Part model, mm, in its own coordinate system. Face numbers are marked on the shaded views. A direction names the side the tool comes from. Round coordinates to 2 decimals unless told otherwise and drop trailing zeros. Write each loop counter-clockwise with the first axis right and the second up, starting at its lowest first coordinate (ties: lowest second). Pieces come first, ordered by that corner, then holes.
1) Pull direction Y, two halves, no side cores. Call the marked faces 3, 4 and 5: +Y half, -Y half, draft (parallel to the pull), parting line (faces both ways), or undercut.
2) Saw through at A-A on y = 0. Write the cut outline in (x, z) (3 decimals).
3) Saw through at D-D on z = -30.5. Write the cut outline in (x, y) (3 decimals), and give its area (3 significant figures).
4) Which spindle directions (+Z, -Z, +X, -X, +Y, -Y) get a long thin tool onto all of the face, cutting with end or side? Do the marked faces 1 and 2. Say none if no direction does.
5) Drill centre lines: L1, parallel to Y at x = 0, z = 8.5 (3 decimals); L2, parallel to Y at x = 0, z = -36 (3 decimals); L3, parallel to Y at x = 1, z = -16. Where is each one in solid material? Low to high.
6) Saw through at B-B on x = 0. Write the cut outline in (y, z) (3 decimals).
7) Flat gauge pins, fed straight in: pin 1 (6 mm diameter, centred on x = 16, z = -18.5, fed in from +Y); pin 2 (10 mm diameter, centred on y = -21, z = -27, fed in from -X); pin 3 (12 mm diameter, centred on y = 50.5, z = -7, fed in from +X); pin 4 (1 mm diameter, centred on y = -29, z = 2, fed in from -X). Where does each tip first touch, or does it go through?
8) Saw through at C-C on y = -21. Write the cut outline in (x, z).
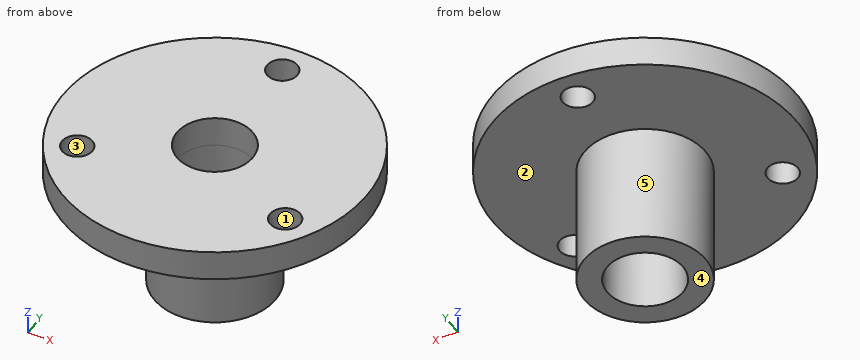
```python
from build123d import *

# Parameters (mm, degrees)
F0_R     = 63.5
F0_R_2   = 6.35
F0_R_3   = 25.4
F0_R_4   = 15.875
F1_DEPTH = 12.7
F2_DEPTH = 50.8


with BuildPart() as f1:
    # F0 (on Top) → F1 (new body)
    with BuildSketch(Plane.XY):
        Circle(F0_R)
        with Locations((-43.994091, -25.4)):
            Circle(F0_R_2, mode=Mode.SUBTRACT)
        with Locations((43.994091, -25.4)):
            Circle(F0_R_2, mode=Mode.SUBTRACT)
        Circle(F0_R_3, mode=Mode.SUBTRACT)
        with Locations((0, 50.8)):
            Circle(F0_R_2, mode=Mode.SUBTRACT)
        Circle(F0_R_3)
        Circle(F0_R_4, mode=Mode.SUBTRACT)
    extrude(amount=F1_DEPTH)

    # F0 (on Top) → F2 (join)
    with BuildSketch(Plane.XY):
        Circle(F0_R_3)
        Circle(F0_R_4, mode=Mode.SUBTRACT)
    extrude(amount=-F2_DEPTH)


solid = f1.part
```
Completed:
1. face 3: undercut
1. face 4: draft
1. face 5: parting line
2. outline: (-63.5, 0) - (-25.4, 0) - (-25.4, -50.8) - (-15.875, -50.8) - (-15.875, 12.7) - (-63.5, 12.7) - close; (15.875, -50.8) - (25.4, -50.8) - (25.4, 0) - (63.5, 0) - (63.5, 12.7) - (15.875, 12.7) - close
3. outline: circle Ø50.8 at (0, 0); hole circle Ø31.75 at (0, 0)
3. area: 1,240 mm2
4. face 1: +Z, -Z
4. face 2: -Z
5. L1: y = -63.5 to -15.875, 15.875 to 44.45, 57.15 to 63.5
5. L2: y = -25.4 to -15.875, 15.875 to 25.4
5. L3: y = -25.38 to -15.84, 15.84 to 25.38
6. outline: (-63.5, 0) - (-25.4, 0) - (-25.4, -50.8) - (-15.875, -50.8) - (-15.875, 12.7) - (-63.5, 12.7) - close; (15.875, -50.8) - (25.4, -50.8) - (25.4, 0) - (44.45, 0) - (44.45, 12.7) - (15.875, 12.7) - close; (57.15, 0) - (63.5, 0) - (63.5, 12.7) - (57.15, 12.7) - close
7. pin 1: stops at y = 21.82
7. pin 2: stops at x = -19.73
7. pin 3: passes through
7. pin 4: stops at x = -56.75
8. outline: (-59.93, 0) - (-48.57, 0) - (-48.57, 12.7) - (-59.93, 12.7) - close; (-39.42, 0) - (-14.29, 0) - (-14.29, -50.8) - (14.29, -50.8) - (14.29, 0) - (39.42, 0) - (39.42, 12.7) - (-39.42, 12.7) - close; (48.57, 0) - (59.93, 0) - (59.93, 12.7) - (48.57, 12.7) - close
